The listing builds one solid part. Answer for the finished solid, in the listing's coordinates (mm). Face numbers are marked on the shaded views. A direction names the side the tool comes from. Give positions to 0.01 mm unless a question says otherwise; leave off trailing zeros. Write each loop counter-clockwise with the first axis right and the second up, starting at its lowest first coordinate (ties: lowest second). Pieces come first, ordered by that corner, then holes. Notation, with made-up numbers: (61.5, 72.5) - (74.5, 72.5) arc R9 cw to (74.5, 83.5) - close; hole circle Ø8 at (26, -21.75). An arc over 180 degrees is marked (long way). Return JSON: item names as keys, results as strings.
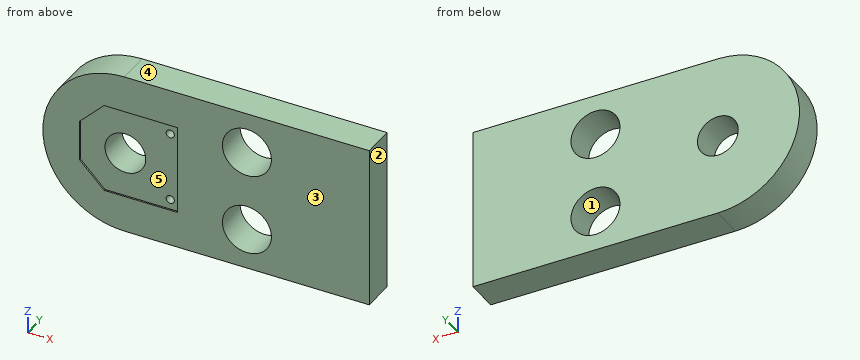
from build123d import *

# Parameters (mm, degrees)
SKETCH1_R           = 2.5
BOSS_EXTRUDE1_DEPTH = 4
CUT_EXTRUDE2_DEPTH  = 0.2
SKETCH6_R           = 0.5
CUT_EXTRUDE3_DEPTH  = 1.5
SKETCH7_R           = 3
CUT_EXTRUDE4_DEPTH  = 32.874754901


with BuildPart() as part:
    # Sketch1 → Boss-Extrude1 (new body)
    with BuildSketch(Plane(origin=(0, 0, 0), x_dir=(1, 0, 0), z_dir=(0, 1, 0))):
        with BuildLine():
            Line((10, 10), (30, 10))
            Line((30, 10), (30, -10))
            Line((30, -10), (10, -10))
            Line((10, -10), (0, -10))
            ThreePointArc((0, -10), (-10, 0), (0, 10))
            Line((0, 10), (10, 10))
        make_face()
        with Locations(Location((0, 0, 0), (0, 0, 270))):
            Circle(SKETCH1_R, mode=Mode.SUBTRACT)
    extrude(amount=BOSS_EXTRUDE1_DEPTH)

    # Sketch5 → Cut-Extrude2 (cut)
    with BuildSketch(Plane.XZ):
        Polygon((-5.5, -2.5), (-5.5, 2.5), (-2.5, 5.5), (6.5, 5.5), (6.5, -5.5), (-2.5, -5.5), align=None)
    extrude(amount=-CUT_EXTRUDE2_DEPTH, mode=Mode.SUBTRACT)

    # Sketch6 → Cut-Extrude3 (cut)
    with BuildSketch(Plane.XZ):
        with Locations(Location((5.5, 4.25, 0), (0, 0, 270))):
            Circle(SKETCH6_R)
        with Locations(Location((5.5, -4.25, 0), (0, 0, 270))):
            Circle(SKETCH6_R)
    extrude(amount=-CUT_EXTRUDE3_DEPTH, mode=Mode.SUBTRACT)

    # Sketch7 → Cut-Extrude4 (cut, through all)
    with BuildSketch(Plane(origin=(0, 4, 0), x_dir=(1, 0, 0), z_dir=(0, 1, 0))):
        with Locations(Location((15, 5, 0), (0, 0, 270))):
            Circle(SKETCH7_R)
        with Locations(Location((15, -5, 0), (0, 0, 270))):
            Circle(SKETCH7_R)
    extrude(amount=-CUT_EXTRUDE4_DEPTH, mode=Mode.SUBTRACT)


solid = part.part
Item 1: A cutting plane is placed at A-A on y = 3.5. Determine the outline of the cut face in (x, z).
Answer below:
{"outline": "(0, -10) - (30, -10) - (30, 10) - (0, 10) arc R10 ccw to start; hole circle Ø5 at (0, 0); hole circle Ø6 at (15, -5); hole circle Ø6 at (15, 5)"}
Item 2: Flat-ended cylindrical pins translate along their axes: P1, Ø3, axis at x = 0, z = 0, coming from the +Y side; P2, Ø0.8, axis at x = 5.5, z = -4, coming from the -Y side. Find the tip coordinate at first contact, or state that the pin passes through.
Answer below:
{"P1": "passes through", "P2": "stops at y = 0.2"}
Item 3: A cutting plane is placed at C-C on x = 12.5. Determine the outline of the cut face in (y, z).
Answer below:
{"outline": "(0, -10) - (4, -10) - (4, -6.66) - (0, -6.66) - close; (0, -3.34) - (4, -3.34) - (4, 3.34) - (0, 3.34) - close; (0, 6.66) - (4, 6.66) - (4, 10) - (0, 10) - close"}
Item 4: Consider L1, parallel to Z at x = 0, y = 2.4; L2, parallel to X at y = 1.1, z = -4.25; L3, parallel to X at y = 0.85, z = 4. Determine where each line is inside the solid, lowest interval first.
Answer below:
{"L1": "z = -10 to -2.5, 2.5 to 10", "L2": "x = -9.05 to 5, 6 to 12.1, 17.9 to 30", "L3": "x = -9.17 to 5.07, 5.93 to 12.17, 17.83 to 30"}
Item 5: The mould has two halves that part along X. Classify the marked faces 1, 2 and 3: +X half, -X half, draft (parallel to the pull), parting line (faces both ways), or undercut.
Answer below:
{"face 1": "undercut", "face 2": "+X half", "face 3": "draft"}
Item 6: A cutting plane is placed at B-B on z = 0. Determine the outline of the cut face in (x, y).
Answer below:
{"outline": "(-10, 0) - (-5.5, 0) - (-5.5, 0.2) - (-2.5, 0.2) - (-2.5, 4) - (-10, 4) - close; (2.5, 0.2) - (6.5, 0.2) - (6.5, 0) - (30, 0) - (30, 4) - (2.5, 4) - close"}
Item 7: For the marked faces 4 and 5, determine the directions among +Z, -Z, +X, -X, +Y, -Y from which every point of the face is accessible in a straight line to the end or side of a thin tool.
Answer below:
{"face 4": "+Z, +X, -X, +Y, -Y", "face 5": "-Y"}
Item 8: A cutting plane is placed at D-D on y = 0.6. Determine the outline of the cut face in (x, z), then the cut area to 3 significant figures.
Answer below:
{"outline": "(0, -10) - (30, -10) - (30, 10) - (0, 10) arc R10 ccw to start; hole circle Ø5 at (0, 0); hole circle Ø1 at (5.5, -4.25); hole circle Ø1 at (5.5, 4.25); hole circle Ø6 at (15, -5); hole circle Ø6 at (15, 5)", "area": "679 mm²"}
